from build123d import *

# Parameters (mm, degrees)
SKETCH1_W      = 720
SKETCH1_H      = 140
SKETCH1_R      = 15.5
EXTRUDE1_DEPTH = 12
SKETCH2_W      = 720
SKETCH2_H      = 12
EXTRUDE2_DEPTH = 126
SKETCH3_R      = 15.5
EXTRUDE3_DEPTH = 168


with BuildPart() as part:
    # Sketch1 → Extrude1 (new body)
    with BuildSketch(Plane.XY):
        with Locations((360, 70)):
            Rectangle(SKETCH1_W, SKETCH1_H)
        with Locations((100, 87)):
            Circle(SKETCH1_R, mode=Mode.SUBTRACT)
        with Locations((200, 87)):
            Circle(SKETCH1_R, mode=Mode.SUBTRACT)
        with Locations((300, 87)):
            Circle(SKETCH1_R, mode=Mode.SUBTRACT)
        with Locations((520, 87)):
            Circle(SKETCH1_R, mode=Mode.SUBTRACT)
        with Locations((620, 87)):
            Circle(SKETCH1_R, mode=Mode.SUBTRACT)
        with Locations((420, 87)):
            Circle(SKETCH1_R, mode=Mode.SUBTRACT)
    extrude(amount=EXTRUDE1_DEPTH)

    # Sketch2 → Extrude2 (add)
    with BuildSketch(Plane.XY.offset(12)):
        with Locations((360, 6)):
            Rectangle(SKETCH2_W, SKETCH2_H)
    extrude(amount=EXTRUDE2_DEPTH)

    # Sketch3 → Extrude3 (cut)
    with BuildSketch(Plane(origin=(0, 12, 0), x_dir=(1, 0, 0), z_dir=(0, 1, 0))):
        with Locations(Location((50, -77, 0), (0, 0, 270))):
            Circle(SKETCH3_R)
        with Locations(Location((150, -77, 0), (0, 0, 270))):
            Circle(SKETCH3_R)
        with Locations(Location((250, -77, 0), (0, 0, 270))):
            Circle(SKETCH3_R)
        with Locations(Location((670, -77, 0), (0, 0, 270))):
            Circle(SKETCH3_R)
        with Locations(Location((470, -77, 0), (0, 0, 270))):
            Circle(SKETCH3_R)
        with Locations(Location((570, -77, 0), (0, 0, 270))):
            Circle(SKETCH3_R)
    extrude(amount=-EXTRUDE3_DEPTH, mode=Mode.SUBTRACT)


solid = part.part
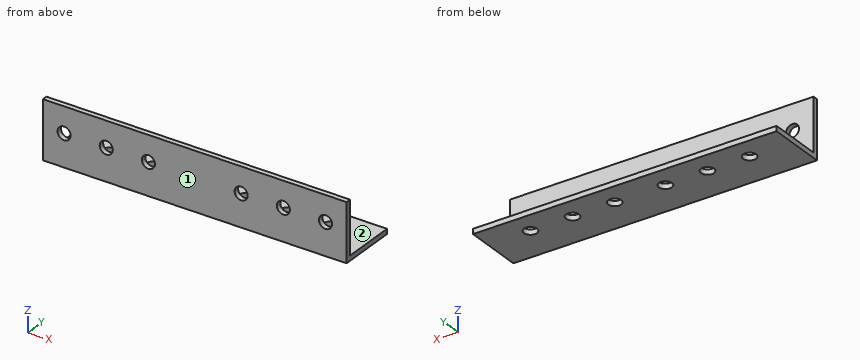
Build history of the part. All positions in model axes, mm. Face numbers are marked on the shaded views. A direction names the side the tool comes from. Coordinates: 2 decimals unless noted, no trailing zeros. Order: outer loops, then holes, each group sorted by start corner. A loop starts at its lowest first (then second) coordinate and runs counter-clockwise, first axis right, second up. Notation, with made-up numbers: M 2.5,-19 L 22.5,-19 A17 cw 22.5,-6 Z; hole C 77,14.5 d4. An arc over 180 degrees is marked long. One line per question, with ' | ' between items. Start each with the question number.
Q1. Saw through at C-C (z = 77). List the corners of the cut face in (x, y), then the cut area to 3 significant figures.
Q2. Flat gauge pins, fed straight in: pin 1 Ø25 at (x, y) = (620, 87) entering from +Z; pin 2 Ø12 at (x, y) = (350.5, 120.5) entering from +Z. Where does each tip first touch, or does it go through?
Q3. Probe L1, parallel to Y at x = 620, z = 7; L2, parallel to Z at x = 210, y = 23. List the from-to ranges inside material, lowest first. Write a range as from..to.
Q4. 3-axis set-ups, long thin cutter, end or side, ignore diameter. For the marked faces 1 and 2: which of +Z, -Z, +X, -X, +Y, -Y reach the whole face in a straight line?
Q5. Saw through at A-A (x = 520). List the corners of the cut face in (y, z), then the cut area to 3 significant figures.
Q6. Saw through at B-B (y = 87). List the corners of the cut face in (x, z).
Q7. Saw through at D-D (y = 35.5). List the corners of the cut face in (x, z), then the cut area to 3 significant figures.
Check values:
1) outline: M 0,0 L 34.5,0 L 34.5,12 L 0,12 Z; M 65.5,0 L 134.5,0 L 134.5,12 L 65.5,12 Z; M 165.5,0 L 234.5,0 L 234.5,12 L 165.5,12 Z; M 265.5,0 L 454.5,0 L 454.5,12 L 265.5,12 Z; M 485.5,0 L 554.5,0 L 554.5,12 L 485.5,12 Z; M 585.5,0 L 654.5,0 L 654.5,12 L 585.5,12 Z; M 685.5,0 L 720,0 L 720,12 L 685.5,12 Z | area: 6,410 mm2
2) pin 1: passes through | pin 2: stops at z = 12
3) L1: y = 0..71.5, 102.5..140 | L2: z = 0..12
4) face 1: +Z, -Z, +X, -X, -Y | face 2: +Z, +X, -X, +Y
5) outline: M 0,0 L 71.5,0 L 71.5,12 L 12,12 L 12,138 L 0,138 Z; M 102.5,0 L 140,0 L 140,12 L 102.5,12 Z | area: 2,820 mm2
6) outline: M 0,0 L 84.5,0 L 84.5,12 L 0,12 Z; M 115.5,0 L 184.5,0 L 184.5,12 L 115.5,12 Z; M 215.5,0 L 284.5,0 L 284.5,12 L 215.5,12 Z; M 315.5,0 L 404.5,0 L 404.5,12 L 315.5,12 Z; M 435.5,0 L 504.5,0 L 504.5,12 L 435.5,12 Z; M 535.5,0 L 604.5,0 L 604.5,12 L 535.5,12 Z; M 635.5,0 L 720,0 L 720,12 L 635.5,12 Z
7) outline: M 0,0 L 720,0 L 720,12 L 0,12 Z | area: 8,640 mm2
